Here's the drawing with two shaded views (mm, measured from the low corner). I have some questions. Coordinates: 2 decimals unless noted, no trailing zeros. Write each loop counter-clockwise with the first axis right and the second up, starting at its lowest first coordinate (ties: lowest second). Pieces come first, ordered by that corner, then holes. Notation, with made-up numbers: M 14.25,27 L 37.25,27 A33 ccw 37.25,60 Z; hole C 46.5,66 d7. An arc over 180 degrees is marked long. Answer as CSV lines item,"result". Start each with the question number.
Item 1: Suppose I cut it at C-C, the plane x = 27.5. Write out the boundary of the cut face in (y, z).
Item 2: Suppose I cut it at D-D, the plane y = 34. Write out the boundary of the cut face in (x, z).
Item 3: Suppose I cut it at A-A, the plane y = 7.5. Write out the boundary of the cut face in (x, z), and give its area (3 significant figures).
Item 4: I'm going to push flat-ended pins straight in: P1, Ø3, axis at x = 20, y = 7.5, coming from the -Z side; P2, Ø0.9, axis at x = 6.5, z = 1, coming from the -Y side; P3, Ø0.9, axis at y = 10, z = 2, coming from the -X side. Where does each tip first touch, or does it pass through?
Item 5: If I drill on line 1 along Y through (x, z) = (27.5, 1.95); line 2 along Y through (x, z) = (12.5, 1.2); line 3 along Y through (x, z) = (24, 0.7), over which ranges is the centre line in solid material (lowest first)? Write a range as [from, to].
Item 6: Suppose I cut it at B-B, the plane z = 1.75. Write out the boundary of the cut face in (x, y).
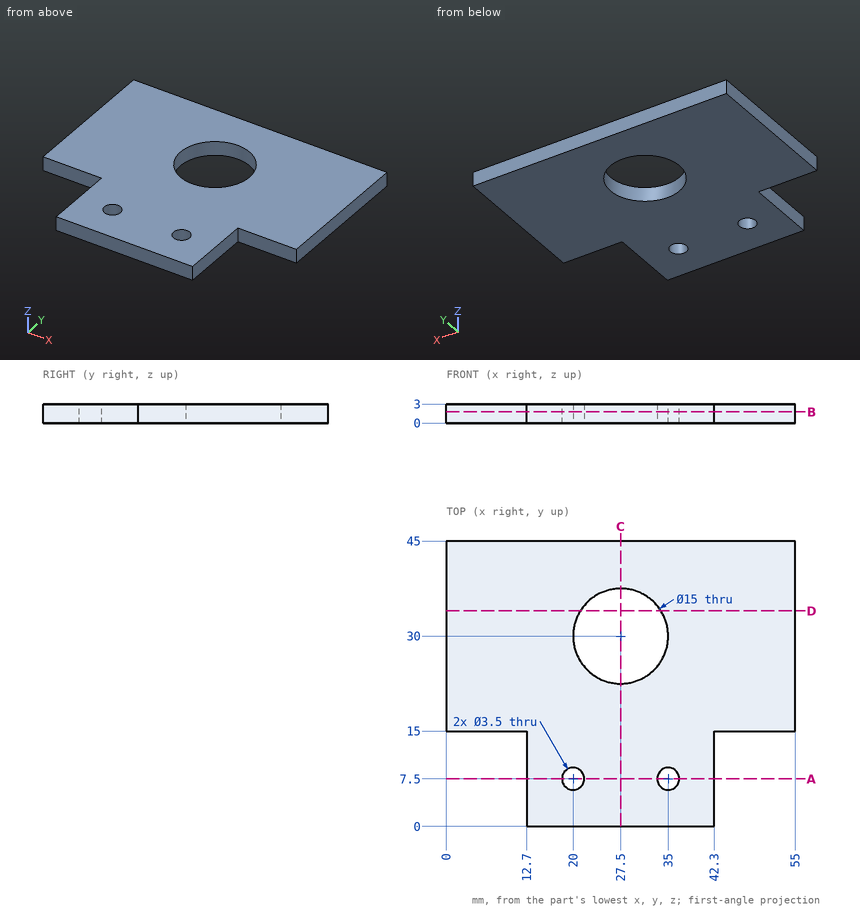
Ans:
1,outline,"M 0,0 L 22.5,0 L 22.5,3 L 0,3 Z; M 37.5,0 L 45,0 L 45,3 L 37.5,3 Z"
2,outline,"M 0,0 L 21.16,0 L 21.16,3 L 0,3 Z; M 33.84,0 L 55,0 L 55,3 L 33.84,3 Z"
3,outline,"M 12.7,0 L 18.25,0 L 18.25,3 L 12.7,3 Z; M 21.75,0 L 33.25,0 L 33.25,3 L 21.75,3 Z; M 36.75,0 L 42.3,0 L 42.3,3 L 36.75,3 Z"
3,area,"67.8 mm^2"
4,P1,"passes through"
4,P2,"stops at y = 15"
4,P3,"stops at x = 12.7"
5,line 1,"y = [0, 22.5], [37.5, 45]"
5,line 2,"y = [15, 45]"
5,line 3,"y = [0, 23.37], [36.63, 45]"
6,outline,"M 0,15 L 12.7,15 L 12.7,0 L 42.3,0 L 42.3,15 L 55,15 L 55,45 L 0,45 Z; hole C 20,7.5 d3.5; hole C 27.5,30 d15; hole C 35,7.5 d3.5"
